Input: part model. Units: mm. Frame: model coordinates. Face numbers are marked on the shaded views. A direction names the side the tool comes from. Round coordinates to 2 decimals unless told otherwise and drop trailing zeros. Loops run counter-clockwise (first coordinate to the right, second up) from the corner with the lowest first, then second, coordinate; pieces in that order, holes last. Notation, with made-up numbers: M -20,41.25 L -3,41.25 A6 ccw -3,48.25 Z; hole C -20.75,36 d1. An arc over 180 degrees is marked long. Return JSON: item names as keys, results as strings. Group by question number.
1) Material intervals for line 1 (Y direction, x = -0.05, z = 3.55) (3 decimals); line 2 (Z direction, x = 1.2, y = 0.5); line 3 (Z direction, x = 1.4, y = -2.5), sorted ascending. Write a range as from..to.
2) Access query for the marked faces 1 and 2. Directions: +Z, -Z, +X, -X, +Y, -Y. A direction counts if a zero-diameter tool reaches every point of the face in a straight line with its end or side. Return the directions, or none.
3) Contact query for flat-ended pins moving along their axis: P1, Ø1, axis at x = 2, y = 1.5, coming from the -Z side; P2, Ø0.6, axis at y = 0, z = 0, coming from the +X side; P3, Ø1.5, axis at x = 2.5, z = 1, coming from the -Y side; P4, Ø1.5, axis at x = 1.5, z = 0.5, coming from the -Y side. Output: stop coordinate, or through.
4) Section B-B (y = 1.5). Output: boundary loops of the cut face in (x, z).
5) Section A-A (x = 2.25). Output: boundary loops of the cut face in (y, z) (3 decimals), plus the area to 3 significant figures.
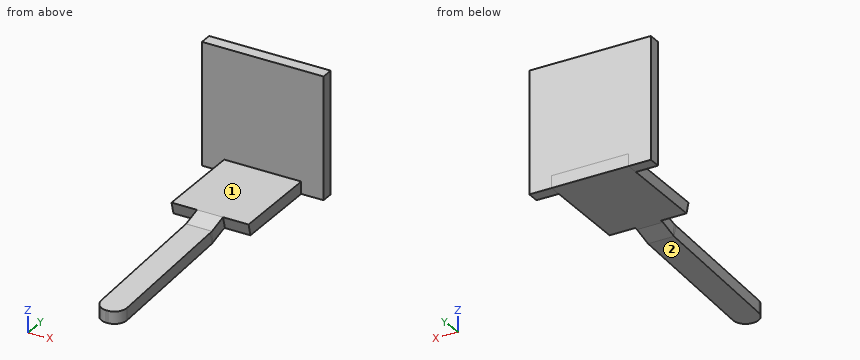
Autodesk Inventor part; units mm, degrees
ref_plane "YZ Plane" through (0, 0, 0) normal (1, 0, 0) x (0, 1, 0)
ref_plane "XZ Plane" through (0, 0, 0) normal (0, 1, 0) x (-1, 0, 0)
ref_plane "XY Plane" through (0, 0, 0) normal (0, 0, 1) x (1, 0, 0)
sketch "Sketch1" plane through (0, 0, 0) normal (0, 0, 1) x (1, 0, 0)
  line L0 (0, 0) -> (2.413, 0)
  line L1 (2.413, 0) -> (2.413, 3.175)
  line L2 (2.413, 3.175) -> (0, 3.175)
  line L3 (0, 3.175) -> (0, 0)
  dimension "d0" = 2.413
  dimension "d1" = 3.175
extrude "Extrusion1" add sketch "Sketch1" along normal blind 0.381
sketch "Sketch2" plane through (2.413, 0, 0) normal (1, 0, 0) x (0, 0, -1)
  line L0 (0, 3.175) -> (-0.381, 3.175)
  line L1 (0, 0) -> (-0.381, 0)
  line L2 (-0.381, 0) -> (-0.2241, -0.5857)
  line L3 (0, 0) -> (0.1569, -0.5857)
  line L4 (-0.2253, -0.5809) -> (0.0185, -5.461)
  line L5 (0.1562, -0.5831) -> (0.3999, -5.461)
  line L6 (-0.381, 0) -> (-0.381, 3.175)
  line L7 (0.0185, -5.461) -> (0.3999, -5.461)
  dimension "d5" = 0.381
  dimension "d6" = 8.636
extrude "Extrusion2" add sketch "Sketch2" against normal up to surface (2.413 mm away)
sketch "Sketch3" plane through (2.413, -5.461, -0.0185) normal (0, -0.0499, 0.9988) x (1, 0, 0)
  line L0 (-2.413, 4.8862) -> (-2.413, 0)
  line L1 (0, 4.8862) -> (-2.413, 4.8862)
  line L2 (-2.413, 5.4741) -> (0, 5.4741)
  line L3 (-2.413, -0.5509) -> (-1.6129, -0.5509)
  line L4 (-1.6129, -0.5509) -> (-1.6129, 4.8862)
  line L5 (-1.6129, 5.4741) -> (-2.413, 5.4741)
  line L6 (-2.413, 4.8862) -> (-2.413, -0.5509)
  line L7 (-0.4584, 5.4741) -> (0, 5.4741)
  line L8 (0, 5.4741) -> (0, 0)
  line L9 (-0.8001, -0.511) -> (0, -0.511)
  line L10 (-0.8001, -0.511) -> (-0.8001, 4.8862)
  line L11 (0, 4.8862) -> (0, -0.511)
  line L12 (-0.8001, 4.8862) -> (0, 4.8862)
  line L13 (-1.6129, 4.8862) -> (-2.413, 4.8862)
  point P0 (-2.413, 5.4551)
  dimension "d9" = 0.8128
  dimension "d10" = 2.413
  dimension "d11" = 0.8001
extrude "Extrusion3" cut sketch "Sketch3" against normal through all
sketch "Sketch4" plane through (0, 0, 0.381) normal (0, -0.2588, 0.9659) x (1, 0, 0)
  line L0 (0, 0) -> (2.413, 0)
  line L1 (1.6129, -0.7023) -> (2.413, -0.7023)
  line L2 (2.413, -0.7023) -> (2.413, 0)
  line L3 (2.413, 0) -> (1.6129, 0)
  line L4 (1.6129, 0) -> (1.6129, -0.7023)
  line L5 (0, -0.7023) -> (0.8001, -0.7023)
  line L6 (0.8001, -0.7023) -> (0.8001, 0)
  line L7 (0.8001, 0) -> (0, 0)
  line L8 (0, 0) -> (0, -0.7023)
  point P0 (0, -0.0986)
extrude "Extrusion4" cut sketch "Sketch4" against normal through all
sketch "Sketch5" plane through (0, 3.175, 0) normal (0, 1, 0) x (1, 0, 0)
  line L0 (2.413, 0) -> (0, 0)
  line L1 (0, 0) -> (0, -0.381)
  line L2 (2.413, -0.381) -> (0, -0.381)
  line L3 (2.413, 0) -> (2.413, -0.381)
  line L4 (-0.6985, 0) -> (3.1115, 0)
  line L5 (3.1115, 0) -> (3.1115, -3.81)
  line L6 (3.1115, -3.81) -> (-0.6985, -3.81)
  line L7 (-0.6985, -3.81) -> (-0.6985, 0)
  dimension "d16" = 3.81
  dimension "d17" = 3.81
  dimension "d18" = 2.413
  dimension "d19" = 0.6985
extrude "Extrusion5" add sketch "Sketch5" against normal blind 0.381 contours L4 L5 L6 L7 L1 L2 L3
fillet "Fillet1" radius 0.381 2 edges at (0.8001, -5.461, -0.2092) (1.6129, -5.461, -0.2092)
equation "\"d11\" = -0.5 * d9 + 0.5 * d10"
equation "\"d19\" = -0.5 * d18 + 0.5 * d16"
properties part number "pin_2"
Returned:
{
 "1": {"line 1": "y = 2.794..3.175", "line 2": "z = 0..0.38", "line 3": "z = -0.25..0.13"},
 "2": {"face 1": "+Z, +X, -X, -Y", "face 2": "-Z, +X, -X, +Y"},
 "3": {"P1": "stops at z = 0", "P2": "stops at x = 2.41", "P3": "stops at y = 0", "P4": "stops at y = -5.46"},
 "4": {"outline": "M 0,0 L 2.41,0 L 2.41,0.38 L 0,0.38 Z"},
 "5": {"outline": "M 0,0.381 L 0.102,0 L 3.175,0 L 3.175,3.81 L 2.794,3.81 L 2.794,0.381 Z", "area": "2.50 mm^2"}
}
